CAD build for the part. Positions are in the model's coordinates, mm. A direction names the side the tool comes from. Coordinates: 2 decimals unless noted, no trailing zeros. Loops run counter-clockwise (first coordinate to the right, second up) from the corner with the lowest first, then second, coordinate; pieces in that order, holes last.
1) Saw through at D-D, the plane z = 2.05. Write the cut outline in (x, y).
2) Wall check: line 1 along X through (y, z) = (-2, -1); line 2 along Y through (x, z) = (-4.75, 0.3); line 3 along X through (y, z) = (-3, 0.9). Give the ranges that are in metal, low to high.
3) Saw through at C-C, the plane x = -8. Write the cut outline in (y, z).
4) Saw through at B-B, the plane y = -2. Write the cut outline in (x, z), and give its area (3 significant figures).
5) Which spindle directions (+Z, -Z, +X, -X, +Y, -Y) get a long thin tool onto all of the face, cutting with end or side? Do faces 5 (the flat face through (7.2, 6, 0)), 6 (the flat face through (-0.29, 6.96, -1.5)), 7 (the flat face through (6.8, 5.4, 0)), 8 (the cylindrical face through (-5.86, -0.99, 0.04)), 9 (the flat face through (-0.29, 6.96, 1.5)). Say none if no direction does.
6) Pin check, flat tips, straight feed: pin 1 Ø1 at (x, y) = (-5, 6) entering from -Z; pin 2 Ø0.7 at (y, z) = (5, 0.5) entering from -X; pin 3 Ø2 at (y, z) = (7, -1) entering from -X; pin 4 Ø2.5 at (x, y) = (-3, 7.5) entering from +Z. Stop position of each tip, or through.
7) Saw through at A-A, the plane z = -0.7. Write the cut outline in (x, y).
8) Two-plate mould, pull along Y, no slides. Class faces 1 (the flat face through (10, 0, 0)), 2 (the flat face through (0, -5, 0)), 3 (the flat face through (-0.712, 7.173, 0.021)), 4 (the cylindrical face through (5.556, -0.735, 0.035)): +Y half, -Y half, draft (parallel to the pull), parting line (faces both ways), or undercut.
```python
from build123d import *

# Parameters (mm, degrees)
BOSS_EXTRUDE1_DEPTH          = 2.5
F_3_0_3_DIAMETER_HOLE1_D     = 3
F_3_0_3_DIAMETER_HOLE1_DEPTH = 5
F_3_0_3_DIAMETER_HOLE1_TIP   = 0.901290929
BOSS_EXTRUDE2_DEPTH          = 1.5


with BuildPart() as part:
    # Sketch1 → Boss-Extrude1 (new, symmetric)
    with BuildSketch(Plane.XY):
        Polygon((-10, 4), (-0.5, 4), (0.5, 5), (10, 5), (10, -5), (-10, -5), align=None)
    extrude(amount=BOSS_EXTRUDE1_DEPTH, both=True)

    # Ø3.0 (3) Diameter Hole1
    with Locations(Plane(origin=(0, 0, -2.5), x_dir=(-1, 0, 0), z_dir=(0, 0, -1))):
        with Locations((-4.75, -2), (4.75, -2)):
            Hole(F_3_0_3_DIAMETER_HOLE1_D / 2, depth=F_3_0_3_DIAMETER_HOLE1_DEPTH)
            with Locations((0, 0, -(F_3_0_3_DIAMETER_HOLE1_DEPTH + F_3_0_3_DIAMETER_HOLE1_TIP / 2))):  # 118° drill point
                Cone(0, F_3_0_3_DIAMETER_HOLE1_D / 2, F_3_0_3_DIAMETER_HOLE1_TIP, mode=Mode.SUBTRACT)

    # Sketch5 → Boss-Extrude2 (add, symmetric)
    with BuildSketch(Plane.XY):
        Polygon((7.2, 5), (7.2, 6.176383421), (-8.849507866, 8.198431348), (-8.899507866, 7.801568652), (6.8, 5.823616579), (6.8, 5), align=None)
    extrude(amount=BOSS_EXTRUDE2_DEPTH, both=True)


solid = part.part
```
Data:
1. outline: (-10, -5) - (10, -5) - (10, 5) - (0.5, 5) - (-0.5, 4) - (-10, 4) - close; hole circle Ø3 at (-4.75, -2); hole circle Ø3 at (4.75, -2)
2. line 1: x = -10 to -6.25, -3.25 to 3.25, 6.25 to 10
2. line 2: y = -5 to -3.5, -0.5 to 4, 7.28 to 7.68
2. line 3: x = -10 to -5.87, -3.63 to 3.63, 5.87 to 10
3. outline: (-5, -2.5) - (4, -2.5) - (4, 2.5) - (-5, 2.5) - close; (7.69, -1.5) - (8.09, -1.5) - (8.09, 1.5) - (7.69, 1.5) - close
4. outline: (-10, -2.5) - (-6.25, -2.5) - (-6.25, 2.5) - (-10, 2.5) - close; (-3.25, -2.5) - (3.25, -2.5) - (3.25, 2.5) - (-3.25, 2.5) - close; (6.25, -2.5) - (10, -2.5) - (10, 2.5) - (6.25, 2.5) - close
4. area: 70.0 mm2
5. face 5: +Z, -Z, +X, +Y
5. face 6: -Z, +X, -X, +Y
5. face 7: +Z, -Z, -X
5. face 8: +Z, -Z
5. face 9: +Z, +X, -X, +Y
6. pin 1: passes through
6. pin 2: stops at x = 0.15
6. pin 3: stops at x = -8.9
6. pin 4: stops at z = 1.5
7. outline: (-10, -5) - (10, -5) - (10, 5) - (7.2, 5) - (7.2, 6.18) - (-8.85, 8.2) - (-8.9, 7.8) - (6.8, 5.82) - (6.8, 5) - (0.5, 5) - (-0.5, 4) - (-10, 4) - close; hole circle Ø3 at (-4.75, -2); hole circle Ø3 at (4.75, -2)
8. face 1: draft
8. face 2: -Y half
8. face 3: +Y half
8. face 4: undercut
